from build123d import *

# Parameters (mm, degrees)
F1_DEPTH = 40
F2_W     = 2
F2_H     = 18
F3_DEPTH = 18
F4_R     = 1.5875
F5_DEPTH = 2.001
F6_R     = 1.5875
F7_DEPTH = 2.001
F8_SIZE  = 1


with BuildPart() as f1:
    # F0 (on Front) → F1 (new body)
    with BuildSketch(Plane.XZ):
        Polygon((-2, 18), (-2, -2), (18, -2), (18, 0), (0, 0), (0, 18), align=None)
    extrude(amount=-F1_DEPTH)

    # F2 (on face) → F3 (join, through all)
    with BuildSketch(Plane.YZ):
        with Locations((1, 9)):
            Rectangle(F2_W, F2_H)
    extrude(amount=F3_DEPTH)

    # F4 (on face) → F5 (cut, through all)
    with BuildSketch(Plane.XY):
        with Locations((9, 12.5)):
            Circle(F4_R)
        with Locations((9, 27.5)):
            Circle(F4_R)
    extrude(amount=-F5_DEPTH, mode=Mode.SUBTRACT)

    # F6 (on face) → F7 (cut, through all)
    with BuildSketch(Plane.YZ):
        with Locations((35, 9)):
            Circle(F6_R)
        with Locations((20, 9)):
            Circle(F6_R)
    extrude(amount=-F7_DEPTH, mode=Mode.SUBTRACT)

    # F8
    f8_edges = [f1.edges().sort_by_distance(p)[0] for p in [
        (-2, 18.4125, 9),
        (-2, 33.4125, 9),
        (7.4125, 27.5, -2),
        (7.4125, 12.5, -2),
    ]]
    chamfer(f8_edges, length=F8_SIZE)


solid = f1.part
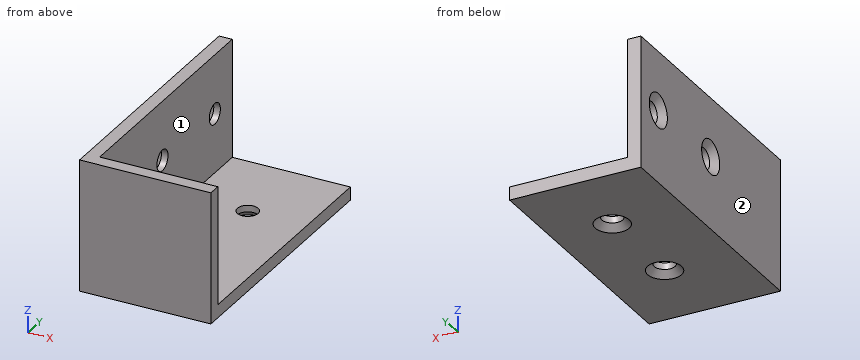
Check sheet for the modelled part. Datum: model origin and axes. Units: mm. Face numbers are marked on the shaded views. A direction names the side the tool comes from. Round coordinates to 2 decimals unless told otherwise and drop trailing zeros. Order: outer loops, then holes, each group sorted by start corner. A loop starts at its lowest first (then second) coordinate and runs counter-clockwise, first axis right, second up.
(1) Cross-section at D-D, the plane x = 5. Enter the section's corners in (y, z), and give its area (3 significant figures).
(2) Go/stop test with flat-tipped pins: P1, Ø2.5, axis at y = 20, z = 9, coming from the -X side; P2, Ø2, axis at x = 7, y = 31, coming from the +Z side; P3, Ø4, axis at y = 35, z = 9, coming from the -X side; P4, Ø3.5, axis at x = 9, y = 12.5, coming from the -Z side. Record where each tip stops, or that it passes through.
(3) Access from +Z, -Z, +X, -X, +Y, -Y to the whole of each face (thin tool, end or side, straight path). Record for the marked faces 1 and 2.
(4) Cross-section at C-C, the plane z = 2.5. Enter the section's corners in (x, y), and give its area (3 significant figures).
(5) Scan lines: probe 1 along Z at (x, y) = (-0.75, 20); probe 2 along Y at (x, z) = (9, -0.5); probe 3 along Y at (x, z) = (3, 0.75). Record each from-to range of solid material in increasing order.
(6) Cross-section at B-B, the plane y = 12.5. Enter the section's corners in (x, z), and give its area (4 significant figures).
(7) Cross-section at A-A, the plane x = 9. Enter the section's corners in (y, z), and give its area (3 significant figures).
Check sheet entries:
1. outline: (0, -2) - (40, -2) - (40, 0) - (2, 0) - (2, 18) - (0, 18) - close
1. area: 116 mm2
2. P1: passes through
2. P2: stops at z = 0
2. P3: stops at x = -1.41
2. P4: stops at z = -1.16
3. face 1: +Z, +X, +Y
3. face 2: +Z, -Z, -X, +Y, -Y
4. outline: (-2, 0) - (18, 0) - (18, 2) - (0, 2) - (0, 40) - (-2, 40) - close
4. area: 116 mm2
5. probe 1: z = -2 to 7.41, 10.59 to 18
5. probe 2: y = 0 to 10.91, 14.09 to 25.91, 29.09 to 40
5. probe 3: y = 0 to 2
6. outline: (-2, -2) - (6.41, -2) - (7.41, -1) - (7.41, 0) - (0, 0) - (0, 18) - (-2, 18) - close; (10.59, -1) - (11.59, -2) - (18, -2) - (18, 0) - (10.59, 0) - close
6. area: 68.65 mm2
7. outline: (0, -2) - (9.91, -2) - (10.91, -1) - (10.91, 0) - (2, 0) - (2, 18) - (0, 18) - close; (14.09, -1) - (15.09, -2) - (24.91, -2) - (25.91, -1) - (25.91, 0) - (14.09, 0) - close; (29.09, -1) - (30.09, -2) - (40, -2) - (40, 0) - (29.09, 0) - close
7. area: 101 mm2
